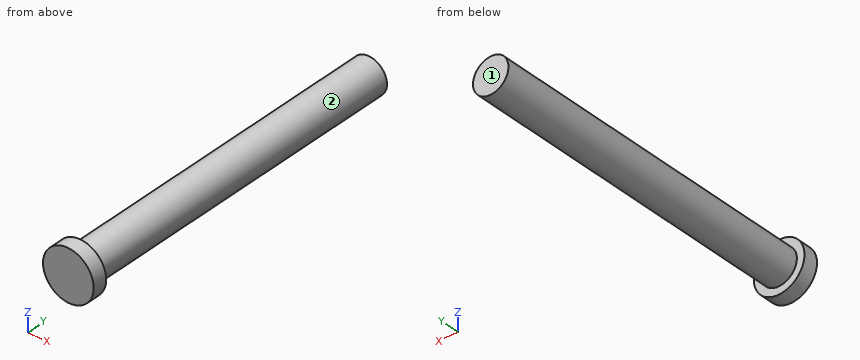
Autodesk Inventor part; units mm, degrees
ref_plane "YZ Plane" through (0, 0, 0) normal (1, 0, 0) x (0, 1, 0)
ref_plane "XZ Plane" through (0, 0, 0) normal (0, 1, 0) x (-1, 0, 0)
ref_plane "XY Plane" through (0, 0, 0) normal (0, 0, 1) x (1, 0, 0)
sketch "Boceto1" plane through (0, 0, 0) normal (0, 1, 0) x (-1, 0, 0)
  circle A0 centre (0, 0) radius 3.5
extrude "Extrusión1" add sketch "Boceto1" against normal blind 2
sketch "Boceto2" plane through (0, 0, 0) normal (0, 1, 0) x (1, 0, 0)
  circle A0 centre (0, 0) radius 2.45
extrude "Extrusión2" add sketch "Boceto2" along normal blind 70
thread "Rosca1"
sketch "Boceto3" plane through (0, 70, 0) normal (0, 1, 0) x (1, 0, 0)
  circle A0 centre (0, 0) radius 2.5
  dimension "d8" = 5
extrude "Extrusión3" cut sketch "Boceto3" against normal blind 25
sketch "Boceto4" plane through (0, 45, 0) normal (0, 1, 0) x (1, 0, 0)
  circle A0 centre (0, 0) radius 2.45
extrude "Extrusión4" add sketch "Boceto4" along normal blind 12
sketch "Boceto5" plane through (0, 57, 0) normal (0, 1, 0) x (1, 0, 0)
  circle A0 centre (0, 0) radius 2.45
extrude "Extrusión5" add sketch "Boceto5" along normal blind 12
sketch "Boceto6" plane through (0, 69, 0) normal (0, 1, 0) x (1, 0, 0)
  circle A0 centre (0, 0) radius 2.45
extrude "Extrusión6" cut sketch "Boceto6" against normal blind 23
properties part number "Tornillo_Corto"
Geometry: final body of the model. Coordinates: model frame, mm. Face numbers are marked on the shaded views. A direction names the side the tool comes from. Round coordinates to 2 decimals unless told otherwise and drop trailing zeros. Order: outer loops, then holes, each group sorted by start corner. A loop starts at its lowest first (then second) coordinate and runs counter-clockwise, first axis right, second up. Notation, with made-up numbers: (54.5, 63.5) -> (87.5, 63.5) arc R26 ccw to (87.5, 86.5) -> close; hole circle Ø9 at (-28.75, 47.5). An arc over 180 degrees is marked (long way). Use one line per item in the form item = value.
(1) Ray query, probe 1 along X at (y, z) = (35, 0); probe 2 along Y at (x, z) = (1.75, -3); probe 3 along X at (y, z) = (17.5, -1.75). Return the intervals inside material, ascending. Write a range as [from, to].
Results list:
probe_1 = [-2.45, 2.45]
probe_2 = [-2, 0]
probe_3 = [-1.71, 1.71]
(2) First-contact query: pin 1 Ø4 at (y, z) = (27, -2.5) entering from -X; pin 2 Ø1.5 at (x, y) = (-1, 36.5) entering from +Z; pin 3 Ø1.5 at (x, y) = (1.5, 31.5) entering from +Z. Flat tips, straight axial feed; report the tip coordinate or a pass-through.
Results list:
pin_1 = -2.4
pin_2 = 2.44
pin_3 = 2.33
(3) Section B-B on x = 0. Return loops of the section in (y, z), and give its area (3 significant figures).
Results list:
outline = (-2, -3.5) -> (0, -3.5) -> (0, -2.45) -> (46, -2.45) -> (46, 2.45) -> (0, 2.45) -> (0, 3.5) -> (-2, 3.5) -> close
area = 239 mm^2
(4) Access query for the marked faces 1 and 2. Directions: +Z, -Z, +X, -X, +Y, -Y. A direction counts if a zero-diameter tool reaches every point of the face in a straight line with its end or side. Return the directions, or none.
Results list:
face_1 = +Z, -Z, +X, -X, +Y
face_2 = +Y
(5) Section D-D on x = 3. Return loops of the section in (y, z).
Results list:
outline = (-2, -1.8) -> (0, -1.8) -> (0, 1.8) -> (-2, 1.8) -> close
(6) Section A-A on z = 0. Return loops of the section in (x, y).
Results list:
outline = (-3.5, -2) -> (3.5, -2) -> (3.5, 0) -> (2.45, 0) -> (2.45, 46) -> (-2.45, 46) -> (-2.45, 0) -> (-3.5, 0) -> close
(7) Section C-C on y = 23. Return loops of the section in (x, z), and give its area (3 significant figures).
Results list:
outline = circle Ø4.9 at (0, 0)
area = 18.9 mm^2
